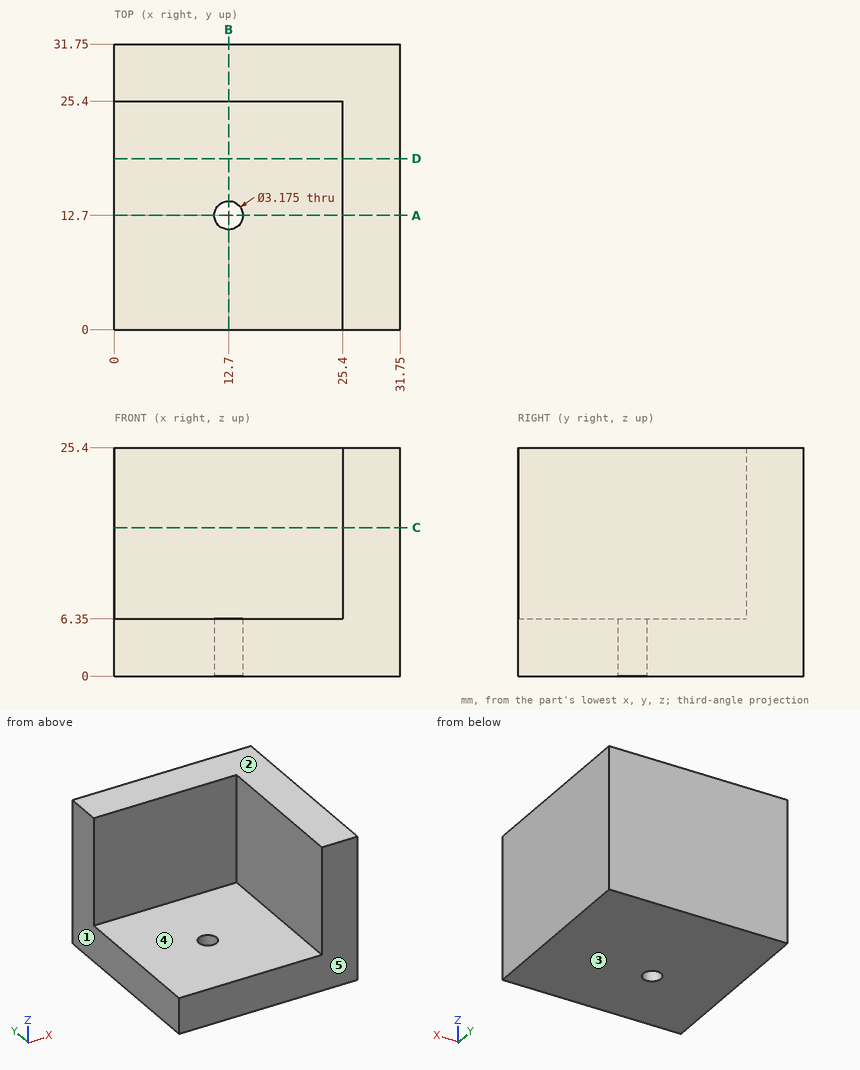
Drawing for the job (mm, zero at the part's lowest x, y, z). A direction names the side the tool comes from. Coordinates: 2 decimals unless noted, no trailing zeros. Order: outer loops, then holes, each group sorted by start corner. A loop starts at its lowest first (then second) coordinate and runs counter-clockwise, first axis right, second up. Notation, with made-up numbers: (-31.5, -30) - (-23.5, -30) arc R14 ccw to (-23.5, -6) - close; hole circle Ø5 at (30, -34.75). An arc over 180 degrees is marked (long way). Use a Markdown table: item, result. Add a question column.
(1) Saw through at D-D (y = 19). Give the cut face in (x, z), then the cut area to 3 significant figures.
(2) Which spindle directions (+Z, -Z, +X, -X, +Y, -Y) get a long thin tool onto all of the face, cutting with end or side? Do the marked faces 4 and 5. Say none if no direction does.
(3) Saw through at C-C (z = 16.5). Give the cut face in (x, y), then the cut area to 3 significant figures.
(4) Saw through at A-A (y = 12.7). Give the cut face in (x, z).
(5) Drill centre lines: line 1 along Y through (x, z) = (12.7, 3.5); line 2 along Z through (x, y) = (13.5, 5.5); line 3 along X through (y, z) = (14.5, 7.75). Where is each one in solid material? Low to high. Write a range as [from, to].
(6) Pull direction Z, two halves, no side cores. Call the marked faces 1, 2 and 3: +Z half, -Z half, draft (parallel to the pull), parting line (faces both ways), or undercut.
(7) Flat gauge pins, fed straight in: pin 1 (5 mm diameter, centred on y = 8.5, z = 19.5, fed in from -X); pin 2 (12.5 mm diameter, centred on x = 10.5, y = 14.5, fed in from +Z); pin 3 (5.5 mm diameter, centred on x = 7.5, z = 13, fed in from -Y). Where does each tip first touch, or does it go through?
Solved:
| question | item | result |
|---|---|---|
| 1 | outline | (0, 0) - (31.75, 0) - (31.75, 25.4) - (25.4, 25.4) - (25.4, 6.35) - (0, 6.35) - close |
| 1 | area | 323 mm² |
| 2 | face 4 | +Z, -X, -Y |
| 2 | face 5 | +Z, -Z, +X, -X, -Y |
| 3 | outline | (0, 25.4) - (25.4, 25.4) - (25.4, 0) - (31.75, 0) - (31.75, 31.75) - (0, 31.75) - close |
| 3 | area | 363 mm² |
| 4 | outline | (0, 0) - (11.11, 0) - (11.11, 6.35) - (0, 6.35) - close; (14.29, 0) - (31.75, 0) - (31.75, 25.4) - (25.4, 25.4) - (25.4, 6.35) - (14.29, 6.35) - close |
| 5 | line 1 | y = [0, 11.11], [14.29, 31.75] |
| 5 | line 2 | z = [0, 6.35] |
| 5 | line 3 | x = [25.4, 31.75] |
| 6 | face 1 | draft |
| 6 | face 2 | +Z half |
| 6 | face 3 | -Z half |
| 7 | pin 1 | stops at x = 25.4 |
| 7 | pin 2 | stops at z = 6.35 |
| 7 | pin 3 | stops at y = 25.4 |
